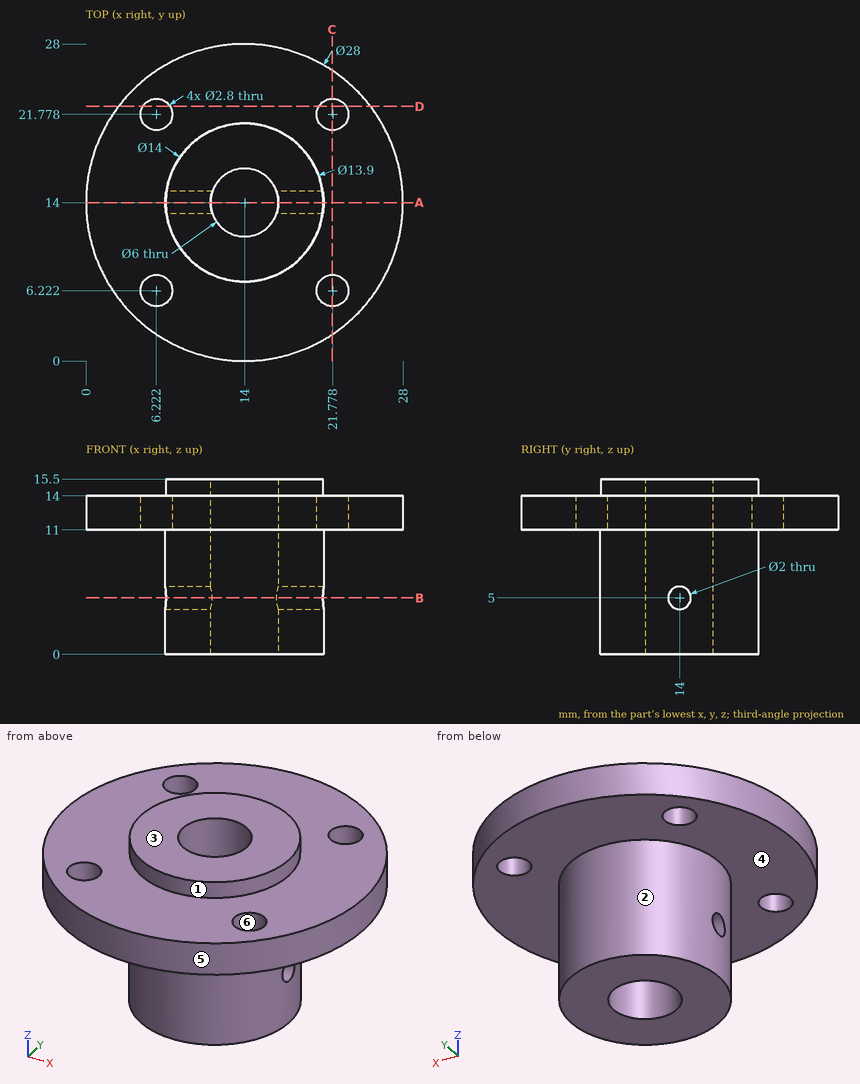
Input: dimensioned drawing with shaded views. Units: mm. Origin: part minimum x, y, z. A direction names the side the tool comes from. Coordinates: 2 decimals unless noted, no trailing zeros. Loops run counter-clockwise (first coordinate to the right, second up) from the corner with the lowest first, then second, coordinate; pieces in that order, holes last. Notation, with made-up numbers: (-15, -21.75) - (10, -21.75) arc R23 ccw to (10, -12.75) - close; hole circle Ø4 at (32.5, 50). An arc over 180 degrees is marked (long way). One line per question, with ' | ' between items. Start each with the question number.
(1) First-contact query: pin 1 (4.5 mm diameter, centred on x = 6.22, y = 21.78, fed in from -Z); pin 2 (1.5 mm diameter, centred on x = 7, z = 13.5, fed in from -Y); pin 3 (6 mm diameter, centred on x = 7.5, z = 7, fed in from +Y). Flat tips, straight axial feed; report the tip coordinate or a pass-through.
(2) Reachability of the marked faces 1, 2 and 3 from +Z, -Z, +X, -X, +Y, -Y: full face, straight path, thin tool, end or side. Return the list, or none.
(3) Ray query, L1, parallel to Z at x = 7.25, y = 19; L2, parallel to X at y = 14.75, z = 1.25 (1 decimal); L3, parallel to Y at x = 14.5, z = 3.25. Return the intervals inside material, ascending. Write a range as from..to.
(4) Draft query along Y for the marked faces 4, 5 and 6. Return one class per face: +Y half, -Y half, draft (parallel to the pull), parting line (faces both ways), or undercut.
(5) Cut plane B-B on z = 5. Output: boundary loops of the cut face in (x, y), and give its area (3 significant figures).
(6) Cut plane C-C on x = 21.75. Output: boundary loops of the cut face in (y, z).
(7) Cut plane D-D on y = 22.5. Output: boundary loops of the cut face in (x, z).
(8) Cut plane A-A on y = 14. Output: boundary loops of the cut face in (x, z), and give its area (3 significant figures).
Here are the results:
1) pin 1: z = 11 | pin 2: y = 1.47 | pin 3: y = 20.06
2) face 1: +Z | face 2: -Z | face 3: +Z, +X, -X, +Y, -Y
3) L1: 11..14 | L2: 7..11.1, 16.9..21 | L3: 7.02..11.04, 16.96..20.98
4) face 4: draft | face 5: parting line | face 6: undercut
5) outline: (7.07, 13) arc R7 ccw to (20.93, 13) - (16.83, 13) arc R3 cw to (11.17, 13) - close; (7.07, 15) - (11.17, 15) arc R3 cw to (16.83, 15) - (20.93, 15) arc R7 ccw to start | area: 110 mm²
6) outline: (2.34, 11) - (4.82, 11) - (4.82, 14) - (2.34, 14) - close; (7.62, 11) - (20.38, 11) - (20.38, 14) - (7.62, 14) - close; (23.18, 11) - (25.66, 11) - (25.66, 14) - (23.18, 14) - close
7) outline: (2.88, 11) - (5.02, 11) - (5.02, 14) - (2.88, 14) - close; (7.42, 11) - (20.58, 11) - (20.58, 14) - (7.42, 14) - close; (22.98, 11) - (25.12, 11) - (25.12, 14) - (22.98, 14) - close
8) outline: (0, 11) - (7, 11) - (7, 6) - (11, 6) - (11, 15.5) - (7.05, 15.5) - (7.05, 14) - (0, 14) - close; (7, 0) - (11, 0) - (11, 4) - (7, 4) - close; (17, 0) - (21, 0) - (21, 4) - (17, 4) - close; (17, 6) - (21, 6) - (21, 11) - (28, 11) - (28, 14) - (20.95, 14) - (20.95, 15.5) - (17, 15.5) - close | area: 150 mm²
